```python
from build123d import *

# Parameters (mm, degrees)
EXTRUDE1_DEPTH      = 2.5
EXTRUDE2_DEPTH      = 5
SKETCH4_R           = 3.05
EXTRUDE4_DEPTH      = 58.470101426
SKETCH5_R           = 2.4
BOSS_EXTRUDE1_DEPTH = 7


with BuildPart() as part:
    # Sketch1 → Extrude1 (new, symmetric)
    with BuildSketch(Plane.XY):
        with BuildLine():
            Line((-14.016148368, -26.524471435), (-4.057181828, -12.697462951))
            ThreePointArc((-4.057181828, -12.697462951), (0, -10.619666847), (4.057181828, -12.697462951))
            Line((4.057181828, -12.697462951), (14.016148368, -26.524471435))
            ThreePointArc((14.016148368, -26.524471435), (0, -53.892923213), (-14.016148368, -26.524471435))
        make_face()
    extrude(amount=EXTRUDE1_DEPTH, both=True)

    # Sketch2 → Extrude2 (add)
    with BuildSketch(Plane(origin=(0, 0, -2.5), x_dir=(-1, 0, 0), z_dir=(0, 0, -1))):
        with BuildLine():
            ThreePointArc((-14.57995219, -27.357357221), (0, -53.892923213), (14.57995219, -27.357357221))
            ThreePointArc((14.57995219, -27.357357221), (0, -31), (-14.57995219, -27.357357221))
        make_face()
    extrude(amount=EXTRUDE2_DEPTH)

    # Sketch4 → Extrude4 (cut, through all)
    with BuildSketch(Plane.XY.offset(2.5)):
        with Locations((0, -36.619666847)):
            Circle(SKETCH4_R)
    extrude(amount=-EXTRUDE4_DEPTH, mode=Mode.SUBTRACT)

    # Sketch5 → Boss-Extrude1 (add)
    with BuildSketch(Plane(origin=(0, 0, -2.5), x_dir=(-1, 0, 0), z_dir=(0, 0, -1))):
        with Locations(Location((0, -15.619666847, 0), (0, 0, 180))):
            Circle(SKETCH5_R)
    extrude(amount=BOSS_EXTRUDE1_DEPTH)


solid = part.part
```
Check sheet for the modelled part. Datum: model origin and axes. Units: mm. A direction names the side the tool comes from. Give positions to 0.01 mm unless a question says otherwise; leave off trailing zeros. Loops run counter-clockwise (first coordinate to the right, second up) from the corner with the lowest first, then second, coordinate; pieces in that order, holes last. Notation, with made-up numbers: M 55.25,-13 L 85.25,-13 A22 cw 85.25,-6 Z; hole C 54,-16 d1. An arc over 180 degrees is marked long. Answer as CSV lines item,"result".
Item 1: Set-up check for faces 4 (the face through (0, -16, -9.5)), 5 (the face through (-0.52, -13.277, -5.951)): record each of +Z, -Z, +X, -X, +Y, -Y from which the full face is reachable in a straight line by a thin tool's end or side.
Reply:
face 4,"-Z, +X, -X, +Y, -Y"
face 5,"-Z"
Item 2: Scan lines: L1, parallel to Z at x = 3, y = -29; L2, parallel to Z at x = -14.5, y = -41; L3, parallel to Y at x = -0.5, z = -0.75. Record each from-to range of solid material in increasing order.
Reply:
L1,"-2.5 to 2.5"
L2,"-7.5 to 2.5"
L3,"-53.89 to -39.63, -33.61 to -10.64"
Item 3: Depth check by flat-ended pin: pin 1 Ø3 at (x, z) = (-1, 0.5) entering from +Y; pin 2 Ø5 at (x, y) = (-1, -41) entering from -Z; pin 3 Ø2 at (x, z) = (-12.5, -4.5) entering from +Y; pin 4 Ø5 at (x, y) = (0, -36.62) entering from +Z. Enter the tip coordinate at first touch or a pass-through.
Reply:
pin 1,"y = -10.62"
pin 2,"z = -7.5"
pin 3,"y = -27.91"
pin 4,"through"
Item 4: Draft check along X on faces 1 (the face through (-9.1, -19.7, 0)), 2 (the face through (1.407, -39.326, -2.43)), 3 (the face through (-0.07, -10.62, 0.04)). Enter one of: pulls with the +X half, pulls with the -X half, needs draft (parallel to the pull), parting line crosses it, or undercut.
Reply:
face 1,"pulls with the -X half"
face 2,"undercut"
face 3,"parting line crosses it"
Item 5: Sectioned sample at A-A, the plane x = 0. Enter the section's corners in (y, z), then the cut area to 3 significant figures.
Reply:
outline,"M -53.89,-7.5 L -39.67,-7.5 L -39.67,2.5 L -53.89,2.5 Z; M -33.57,-7.5 L -31,-7.5 L -31,-2.5 L -18.02,-2.5 L -18.02,-9.5 L -13.22,-9.5 L -13.22,-2.5 L -10.62,-2.5 L -10.62,2.5 L -33.57,2.5 Z"
area,"303 mm^2"
Item 6: Sectioned sample at B-B, the plane y = -30. Enter the section's corners in (x, z).
Reply:
outline,"M -15.95,-7.5 L -7.81,-7.5 L -7.81,-2.5 L 7.81,-2.5 L 7.81,-7.5 L 15.95,-7.5 L 15.95,2.5 L -15.95,2.5 Z"
Item 7: Sectioned sample at C-C, the plane x = -6. Enter the section's corners in (y, z), then the cut area to 3 significant figures.
Reply:
outline,"M -52.82,-7.5 L -30.41,-7.5 L -30.41,-2.5 L -15.39,-2.5 L -15.39,2.5 L -52.82,2.5 Z"
area,"299 mm^2"
Item 8: Sectioned sample at D-D, the plane z = 1.25. Enter the section's corners in (x, y), then the cut area to 3 significant figures.
Reply:
outline,"M -14.02,-26.52 A17.27 ccw long 14.02,-26.52 L 4.06,-12.7 A5 ccw -4.06,-12.7 Z; hole C 0,-36.62 d6.1"
area,"1,030 mm^2"
